Read the model definition and answer for the solid it produces. Units are mm, in the model's axes. A direction names the side the tool comes from. Round coordinates to 2 decimals unless told otherwise and drop trailing zeros. Loops run counter-clockwise (first coordinate to the right, second up) from the corner with the lowest first, then second, coordinate; pieces in that order, holes last. Notation, with made-up numbers: M -29,21.5 L 29,21.5 A25 cw 29,53.5 Z; hole C 87,1.25 d2. An arc over 180 degrees is marked long. Answer as CSV lines item,"result".
```python
from build123d import *

# Parameters (mm, degrees)
SKETCH1_W           = 23
SKETCH1_H           = 12
BOSS_EXTRUDE1_DEPTH = 15.6
SKETCH2_R           = 0.75
BOSS_EXTRUDE2_DEPTH = 1
SKETCH3_R           = 1
SKETCH3_R_2         = 0.5
SKETCH3_R_3         = 0.65
CUT_EXTRUDE1_DEPTH  = 4


with BuildPart() as part:
    # Sketch1 → Boss-Extrude1 (new body)
    with BuildSketch(Plane(origin=(0, 0, 0), x_dir=(1, 0, 0), z_dir=(0, 1, 0))):
        Rectangle(SKETCH1_W, SKETCH1_H)
    extrude(amount=BOSS_EXTRUDE1_DEPTH)

    # Sketch2 → Boss-Extrude2 (add)
    with BuildSketch(Plane(origin=(0, 15.6, 0), x_dir=(1, 0, 0), z_dir=(0, 1, 0))):
        with Locations(Location((-10.2, 4.7, 0), (0, 0, 270))):
            Circle(SKETCH2_R)
        with Locations(Location((10.2, 4.7, 0), (0, 0, 90))):
            Circle(SKETCH2_R)
        with Locations(Location((10.2, -4.7, 0), (0, 0, 270))):
            Circle(SKETCH2_R)
        with Locations(Location((-10.2, -4.7, 0), (0, 0, 90))):
            Circle(SKETCH2_R)
    extrude(amount=BOSS_EXTRUDE2_DEPTH)

    # Sketch3 → Cut-Extrude1 (cut)
    with BuildSketch(Plane(origin=(0, 15.6, 0), x_dir=(1, 0, 0), z_dir=(0, 1, 0))):
        with Locations(Location((6, 0, 0), (0, 0, 270))):
            Circle(SKETCH3_R)
        with Locations(Location((0.5, 0, 0), (0, 0, 270))):
            Circle(SKETCH3_R_2)
        with Locations(Location((-5.5, 0, 0), (0, 0, 270))):
            Circle(SKETCH3_R_3)
    extrude(amount=-CUT_EXTRUDE1_DEPTH, mode=Mode.SUBTRACT)


solid = part.part
```
1) Find section C-C, the plane x = -5.5. Give the vertices of the cut face in (y, z).
Evaluation:
outline,"M 0,-6 L 15.6,-6 L 15.6,-0.65 L 11.6,-0.65 L 11.6,0.65 L 15.6,0.65 L 15.6,6 L 0,6 Z"
2) Find section B-B, the plane x = -10.2. Give the vertices of the cut face in (y, z), then the cut area to 3 significant figures.
Evaluation:
outline,"M 0,-6 L 15.6,-6 L 15.6,-5.45 L 16.6,-5.45 L 16.6,-3.95 L 15.6,-3.95 L 15.6,3.95 L 16.6,3.95 L 16.6,5.45 L 15.6,5.45 L 15.6,6 L 0,6 Z"
area,"190 mm^2"
3) Straight lines are drawn through the part: line 1 (X direction, y = 14, z = 0); line 2 (Y direction, x = 1, z = -4.5). For each, find the intervals that lie inside material, in ascending order.
Evaluation:
line 1,"x = -11.5 to -6.15, -4.85 to 0, 1 to 5, 7 to 11.5"
line 2,"y = 0 to 15.6"
4) Find section A-A, the plane z = 0. Give the vertices of the cut face in (x, y), then the cut area to 3 significant figures.
Evaluation:
outline,"M -11.5,0 L 11.5,0 L 11.5,15.6 L 7,15.6 L 7,11.6 L 5,11.6 L 5,15.6 L 1,15.6 L 1,11.6 L 0,11.6 L 0,15.6 L -4.85,15.6 L -4.85,11.6 L -6.15,11.6 L -6.15,15.6 L -11.5,15.6 Z"
area,"342 mm^2"
5) Find section D-D, the plane z = -4.7. Give the vertices of the cut face in (x, y).
Evaluation:
outline,"M -11.5,0 L 11.5,0 L 11.5,15.6 L 10.95,15.6 L 10.95,16.6 L 9.45,16.6 L 9.45,15.6 L -9.45,15.6 L -9.45,16.6 L -10.95,16.6 L -10.95,15.6 L -11.5,15.6 Z"
6) Determine the mould class of faces 1 (the flat face through (-10, 16.6, 5)), 2 (the flat face through (-11.5, 8, 0)), 3 (the cylindrical face through (7, 14, 0)) for opening direction X: released by +X, released by -X, zero draft, split by the parting line, or undercut.
Evaluation:
face 1,"zero draft"
face 2,"released by -X"
face 3,"undercut"
7) A tool of negligible diameter and unlimited length cuts with its end or side. For faces 4 (the cylindrical face through (-9.568, 16.093, -4.297)), 5 (the flat face through (10, 16.6, -5)), from which of +Z, -Z, +X, -X, +Y, -Y can it reach the whole face along a straight path? Write none if from no direction.
Evaluation:
face 4,"+Y"
face 5,"+Z, -Z, +X, -X, +Y"
8) Each of these flat-tipped pins is pushed along its axis until it touches: P1, Ø1.8, axis at x = 6, z = 0, coming from the +Y side; P2, Ø2, axis at x = -5.5, z = 0, coming from the +Y side. Where does it stop, or does it pass through?
Evaluation:
P1,"stops at y = 11.6"
P2,"stops at y = 15.6"
